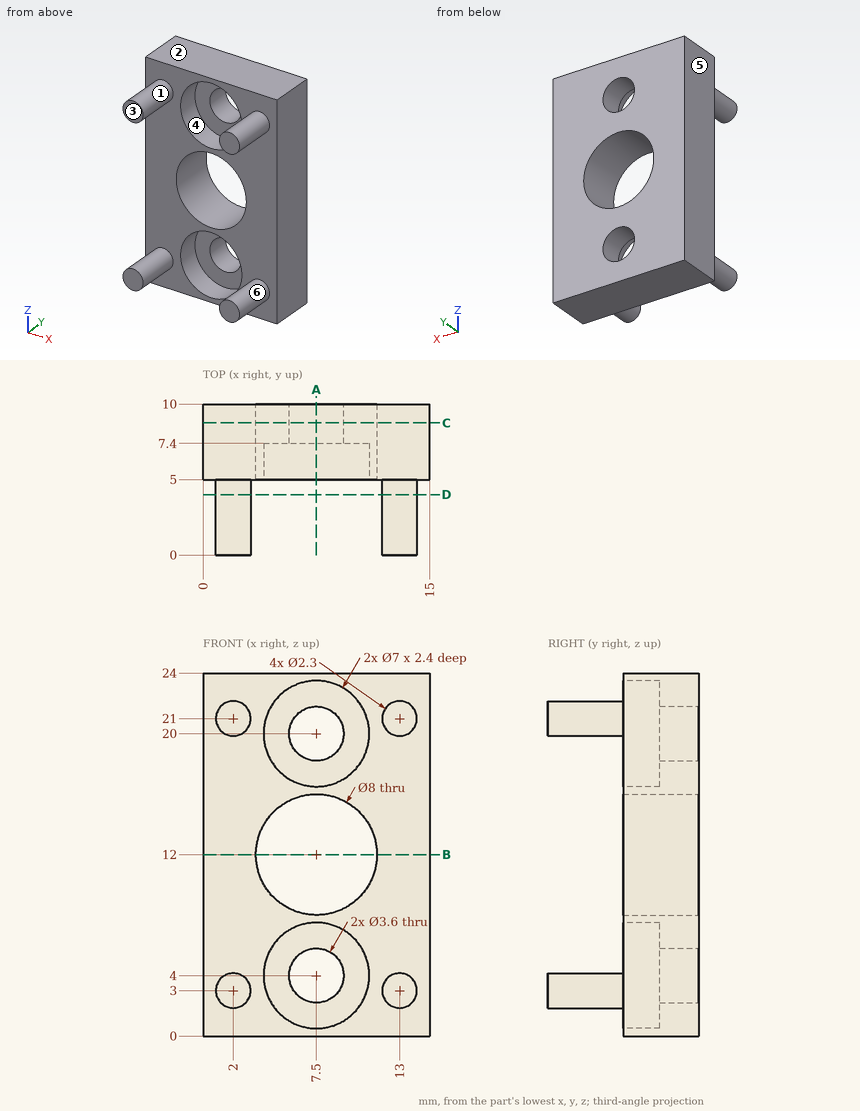
The figure shows three views and two pictorial views of one solid part (mm, origin at its lowest corner). Answer the questions. A direction names the side the tool comes from. Give positions to 0.01 mm unless a question says otherwise; leave off trailing zeros. Order: outer loops, then holes, each group sorted by start corner. A loop starts at its lowest first (then second) coordinate and runs counter-clockwise, first axis right, second up. Notation, with made-up numbers: (69.5, -40) -> (90.5, -40) arc R30 ccw to (90.5, -7) -> close; hole circle Ø1 at (-27.5, -30.5). An arc over 180 degrees is marked (long way). One line per item, written item: value.
1) A tool of negligible diameter and unlimited length cuts with its end or side. For the marked faces 5 and 6, from which of +Z, -Z, +X, -X, +Y, -Y can it reach the whole face along a straight path? Write none if from no direction.
Reported:
face 5: +Z, -Z, -X, +Y, -Y
face 6: -Y
2) Find section A-A, the plane x = 7.5. Determine the outline of the cut face in (y, z).
Reported:
outline: (5, 0) -> (10, 0) -> (10, 2.2) -> (7.4, 2.2) -> (7.4, 0.5) -> (5, 0.5) -> close; (5, 7.5) -> (7.4, 7.5) -> (7.4, 5.8) -> (10, 5.8) -> (10, 8) -> (5, 8) -> close; (5, 16) -> (10, 16) -> (10, 18.2) -> (7.4, 18.2) -> (7.4, 16.5) -> (5, 16.5) -> close; (5, 23.5) -> (7.4, 23.5) -> (7.4, 21.8) -> (10, 21.8) -> (10, 24) -> (5, 24) -> close
3) Flat-ended cylindrical pins translate along their axes: P1, Ø6, axis at x = 9.5, z = 11.5, coming from the -Y side; P2, Ø6.5, axis at x = 7.5, z = 12, coming from the +Y side. Find the tip coordinate at first contact, or state that the pin passes through.
Reported:
P1: stops at y = 5
P2: passes through
4) Find section B-B, the plane z = 12. Determine the outline of the cut face in (x, y).
Reported:
outline: (0, 5) -> (3.5, 5) -> (3.5, 10) -> (0, 10) -> close; (11.5, 5) -> (15, 5) -> (15, 10) -> (11.5, 10) -> close
5) Determine the mould class of the marked faces 1, 2, 3 and 4 for opening direction Z: pulls with the +Z half, pulls with the -Z half, needs draft (parallel to the pull), parting line crosses it, or undercut.
Reported:
face 1: undercut
face 2: pulls with the +Z half
face 3: needs draft
face 4: undercut
6) Find section D-D, the plane y = 4. Determine the outline of the cut face in (x, z).
Reported:
outline: circle Ø2.3 at (2, 3); circle Ø2.3 at (2, 21); circle Ø2.3 at (13, 3); circle Ø2.3 at (13, 21)
7) Find section C-C, the plane y = 8.75. Determine the outline of the cut face in (x, z).
Reported:
outline: (0, 0) -> (15, 0) -> (15, 24) -> (0, 24) -> close; hole circle Ø8 at (7.5, 12); hole circle Ø3.6 at (7.5, 4); hole circle Ø3.6 at (7.5, 20)
8) Find the intervals of material crossed by line 1 (Z direction, x = 7.5, y = 5.9); line 2 (Z direction, x = 7.5, y = 9.3); line 3 (X direction, y = 6.4, z = 20), in increasing order.
Reported:
line 1: z = 0 to 0.5, 7.5 to 8, 16 to 16.5, 23.5 to 24
line 2: z = 0 to 2.2, 5.8 to 8, 16 to 18.2, 21.8 to 24
line 3: x = 0 to 4, 11 to 15
